Here's the drawing with two shaded views (mm, measured from the low corner). I have some questions. Coordinates: 2 decimals unless noted, no trailing zeros. Order: outer loops, then holes, each group sorted by start corner. A loop starts at its lowest first (then second) coordinate and runs counter-clockwise, first axis right, second up. Notation, with made-up numbers: (16.5, -28.5) -> (26.5, -28.5) arc R9 cw to (26.5, -23.5) -> close; hole circle Ø5 at (24, 46). An arc over 180 degrees is marked (long way). Answer in a Markdown table with one row per item. Add a question column.
1. If I drill on line 1 along X through (y, z) = (76.5, 292.1) (3 decimals); line 2 along Z through (x, y) = (292, 42); line 3 along Z through (x, y) = (290, 47.5), over which ranges is the centre line in solid material (lowest first)? Write a range as [from, to].
2. Will these pins go through, and if not, where does the flat tip stop? pin 1 (10 mm diameter, centred on x = 469.5, y = 69.5, fed in from -Z); pin 2 (6 mm diameter, centred on x = 402.5, y = 79.5, fed in from +Z); pin 3 (6 mm diameter, centred on x = 380, z = 189, fed in from -Y); pin 4 (4 mm diameter, centred on y = 76.5, z = 486.5, fed in from -X).
3. Imagine slicing it at A-A on z = 292.1. Write out the boundary of the cut face in (x, y) (3 decimals), plus the area to 3 significant figures.
4. Imagine slicing it at B-B on y = 56. Write out the boundary of the cut face in (x, z) (3 decimals).
5. Imagine slicing it at C-C on y = 11.5. Write out the boundary of the cut face in (x, z) (3 decimals), plus the area to 3 significant figures.
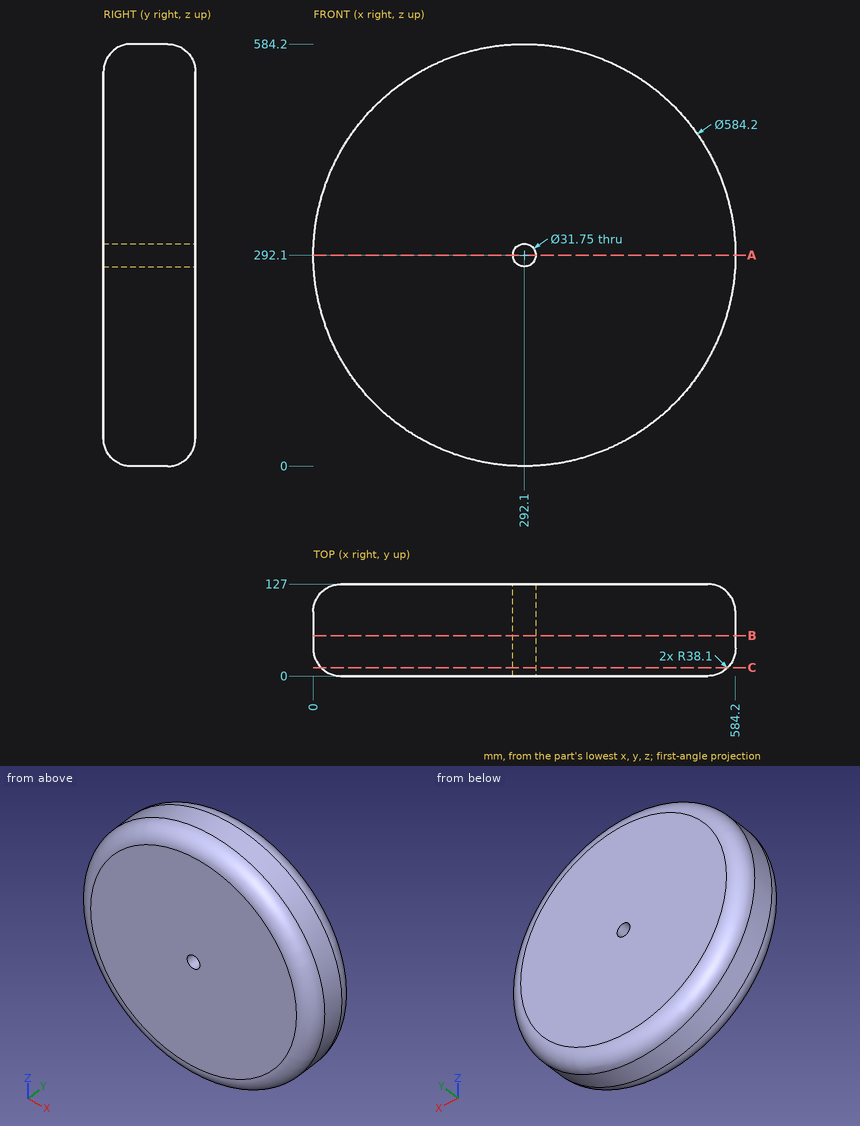
Answers follow:
| question | item | result |
|---|---|---|
| 1 | line 1 | x = [0, 276.225], [307.975, 584.2] |
| 1 | line 2 | z = [0, 276.23], [307.97, 584.2] |
| 1 | line 3 | z = [0.01, 276.36], [307.84, 584.19] |
| 2 | pin 1 | stops at z = 56.3 |
| 2 | pin 2 | stops at z = 563.74 |
| 2 | pin 3 | stops at y = 0 |
| 2 | pin 4 | stops at x = 72.32 |
| 3 | outline | (0, 38.1) arc R38.1 ccw to (38.1, 0) -> (276.225, 0) -> (276.225, 127) -> (38.1, 127) arc R38.1 ccw to (0, 88.9) -> close; (307.975, 0) -> (546.1, 0) arc R38.1 ccw to (584.2, 38.1) -> (584.2, 88.9) arc R38.1 ccw to (546.1, 127) -> (307.975, 127) -> close |
| 3 | area | 68,900 mm² |
| 4 | outline | circle Ø584.2 at (292.1, 292.1); hole circle Ø31.75 at (292.1, 292.1) |
| 5 | outline | circle Ø562.555 at (292.1, 292.1); hole circle Ø31.75 at (292.1, 292.1) |
| 5 | area | 248,000 mm² |
